Design review of the part shown in the three views and the two pictorial views. Dimensions are in mm from the part's minimum x, y and z. Round coordinates to 2 decimals unless told otherwise and drop trailing zeros. Write each loop counter-clockwise with the first axis right and the second up, starting at its lowest first coordinate (ties: lowest second). Pieces come first, ordered by that corner, then holes. Notation, with made-up numbers: (53.25, -23.75) - (79.25, -23.75) arc R21 cw to (79.25, 11.25) - close; hole circle Ø1 at (79, 26.25). An arc over 180 degrees is marked (long way). Use one line per item in the form item = value.
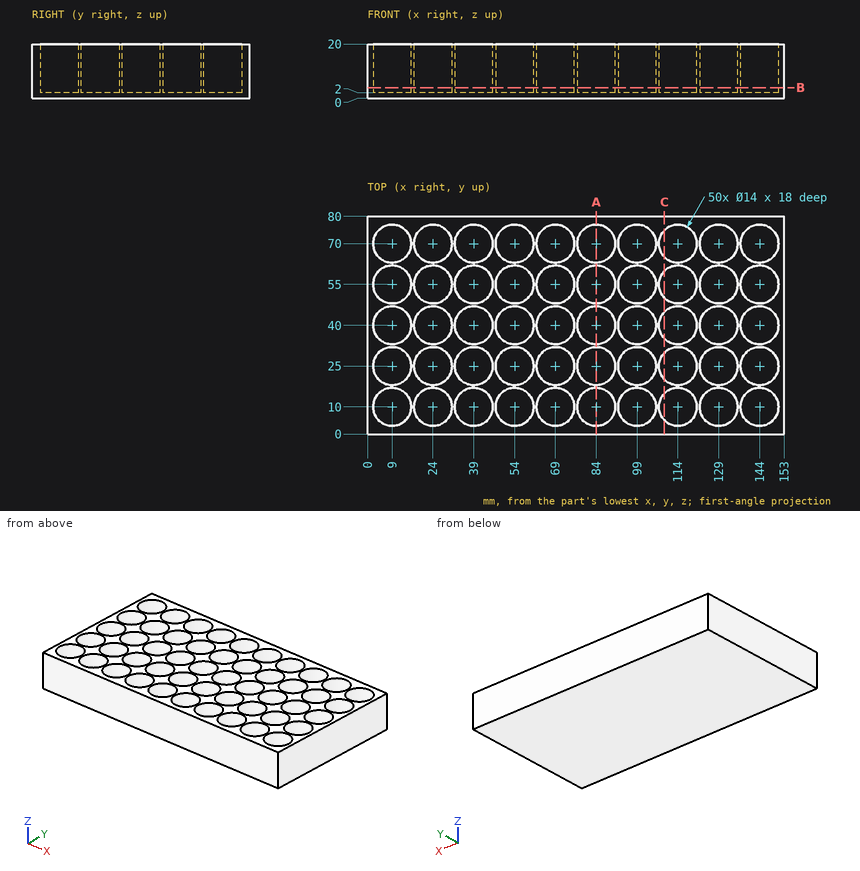
Q1. We need section B-B on z = 4. State how many separate pieces and enclosed holes the cut face has, then the cut area to 3 significant figures.
Calculated:
separate_pieces = 1
enclosed_holes = 50
area = 4,540 mm2
Q2. We need section C-C on x = 109. Write out the cut boundary in (y, z).
Calculated:
outline = (0, 0) - (80, 0) - (80, 20) - (74.9, 20) - (74.9, 2) - (65.1, 2) - (65.1, 20) - (59.9, 20) - (59.9, 2) - (50.1, 2) - (50.1, 20) - (44.9, 20) - (44.9, 2) - (35.1, 2) - (35.1, 20) - (29.9, 20) - (29.9, 2) - (20.1, 2) - (20.1, 20) - (14.9, 20) - (14.9, 2) - (5.1, 2) - (5.1, 20) - (0, 20) - close
Q3. To check wall thickness, follow line 1 along Y through (x, z) = (129, 11); line 2 along Y through (x, z) = (15, 13.75); line 3 along Z through (x, y) = (9, 56.5). State the ranges of each line that lie inside material, in increasing order. Write a range as from..to.
Calculated:
line_1 = 0..3, 17..18, 32..33, 47..48, 62..63, 77..80
line_2 = 0..6.39, 13.61..21.39, 28.61..36.39, 43.61..51.39, 58.61..66.39, 73.61..80
line_3 = 0..2
Q4. We need section A-A on x = 84. Write out the cut boundary in (y, z).
Calculated:
outline = (0, 0) - (80, 0) - (80, 20) - (77, 20) - (77, 2) - (63, 2) - (63, 20) - (62, 20) - (62, 2) - (48, 2) - (48, 20) - (47, 20) - (47, 2) - (33, 2) - (33, 20) - (32, 20) - (32, 2) - (18, 2) - (18, 20) - (17, 20) - (17, 2) - (3, 2) - (3, 20) - (0, 20) - close
Q5. For P1, Ø4, axis at x = 42, y = 9, coming from the +Z side, flat-tipped, find the tip position at first contact; note if it passes through.
Calculated:
P1 = 2
